```python
from build123d import *

# Parameters (mm, degrees)
F0_R     = 45
F0_R_2   = 40
F2_DEPTH = 3
F5_D     = 3
F6_R     = 0.75
F7_DEPTH = 50


with BuildPart() as f2:
    # F0 (on Top) → F2 (new body)
    with BuildSketch(Plane.XY):
        Circle(F0_R)
        Circle(F0_R_2, mode=Mode.SUBTRACT)
    extrude(amount=F2_DEPTH)

    # F5 (through all)
    with Locations(Plane.XY.offset(3)):
        with Locations((-30.052038, 30.052038), (-30.052038, -30.052038), (30.052038, -30.052038), (30.052038, 30.052038)):
            Hole(F5_D / 2)

    # F6 (on Front) → F7 (cut, symmetric)
    with BuildSketch(Plane.XZ):
        with Locations((-25, 1.5)):
            Circle(F6_R)
        with Locations((0, 1.5)):
            Circle(F6_R)
        with Locations((25, 1.5)):
            Circle(F6_R)
    extrude(amount=F7_DEPTH, both=True, mode=Mode.SUBTRACT)


solid = f2.part
```
CAD build for the part. Positions are in the model's coordinates, mm. Round coordinates to 2 decimals unless told otherwise and drop trailing zeros. Loops run counter-clockwise (first coordinate to the right, second up) from the corner with the lowest first, then second, coordinate; pieces in that order, holes last. Notation, with made-up numbers: M 15.5,-35.5 L 43.5,-35.5 A23 cw 43.5,3.5 Z; hole C 63.5,89.25 d1. An arc over 180 degrees is marked long. Return JSON: item names as keys, results as strings. Group by question number.
(1) Wall check: probe 1 along Y at (x, z) = (0, 2.7); probe 2 along X at (y, z) = (34, 1.65); probe 3 along X at (y, z) = (-34.5, 1.25). Give the ranges that are in metal, low to high. Write a range as [from, to].
(2) Drop flat-ended pins along their axis: P1, Ø1.5, axis at x = -31, y = 33, coming from the -Z side; P2, Ø1, axis at y = -27, z = 2, coming from the -X side. Give the stop position or say it passes through.
(3) Mould opens along Y. For faces 1 (the cylindrical face through (-30.86, -28.79, 1.48)), 2 (the cylindrical face through (20.765, -39.923, 1.479)), 3 (the flat face through (-27, 30, 3)), 4 (the cylindrical face through (29.246, -28.787, 1.479)) say: +Y half, -Y half, draft (parallel to the pull), parting line (faces both ways), or undercut.
(4) Saw through at A-A, the plane y = 0. List the corners of the cut face in (x, z), and give its area (3 significant figures).
(5) Saw through at B-B, the plane z = 1.5. Give the number of separate pieces and of enclosed holes in the cut face, and give its area (3 significant figures).
(6) Saw through at C-C, the plane x = -17. List the corners of the cut face in (y, z), and give its area (3 significant figures).
Answer list:
{
 "1": {"probe 1": "[-45, -40], [40, 45]", "probe 2": "[-29.48, -25.73], [-24.27, -21.07], [21.07, 24.27], [25.73, 29.48]", "probe 3": "[-28.89, -25.71], [-24.29, -20.24], [20.24, 24.29], [25.71, 28.89]"},
 "2": {"P1": "z = 0", "P2": "x = -36.37"},
 "3": {"face 1": "undercut", "face 2": "parting line", "face 3": "draft", "face 4": "undercut"},
 "4": {"outline": "M -45,0 L -40,0 L -40,3 L -45,3 Z; M 40,0 L 45,0 L 45,3 L 40,3 Z", "area": "30.0 mm2"},
 "5": {"separate pieces": "6", "enclosed holes": "4", "area": "1,250 mm2"},
 "6": {"outline": "M -41.67,0 L -36.21,0 L -36.21,3 L -41.67,3 Z; M 36.21,0 L 41.67,0 L 41.67,3 L 36.21,3 Z", "area": "32.7 mm2"}
}
